from build123d import *

# Parameters (mm, degrees)
SKETCH_2_W      = 56
SKETCH_2_H      = 32
EXTRUDE_1_DEPTH = 3
SKETCH_3_W      = 56
SKETCH_3_H      = 32
SKETCH_3_W_2    = 25
SKETCH_3_H_2    = 14
EXTRUDE_2_DEPTH = 1
SKETCH_4_R      = 2.4
EXTRUDE_3_DEPTH = 5
SKETCH_6_W      = 56
SKETCH_6_H      = 2
EXTRUDE_4_DEPTH = 4
SKETCH_7_R      = 0.8
EXTRUDE_5_DEPTH = 5


with BuildPart() as part:
    # 草图2 → 凸台-拉伸1 (new body)
    with BuildSketch(Plane(origin=(0, 0, 0), x_dir=(1, 0, 0), z_dir=(0, 1, 0))):
        with Locations((6.832, -6.328)):
            Rectangle(SKETCH_2_W, SKETCH_2_H)
        Polygon((-20.168, -11.589207904), (-20.168, 4.317392289), (-20.168, 8.672), (33.832, 8.672), (33.832, -14.328), (20.832, -14.328), (20.832, -21.328), (-7.168, -21.328), (-7.168, -14.328), (-20.168, -14.328), align=None, mode=Mode.SUBTRACT)
    extrude(amount=EXTRUDE_1_DEPTH)

    # 草图3 → 凸台-拉伸2 (add)
    with BuildSketch(Plane(origin=(0, 3, 0), x_dir=(1, 0, 0), z_dir=(0, 1, 0))):
        with Locations((6.832, -6.328)):
            Rectangle(SKETCH_3_W, SKETCH_3_H)
        with Locations((6.832, -5.328)):
            Rectangle(SKETCH_3_W_2, SKETCH_3_H_2, mode=Mode.SUBTRACT)
    extrude(amount=EXTRUDE_2_DEPTH)

    # 草图4 → 凸台-拉伸3 (add)
    with BuildSketch(Plane(origin=(0, 0, 0), x_dir=(-1, 0, 0), z_dir=(0, -1, 0))):
        with Locations(Location((16.168, -18.328, 0), (0, 0, 270))):
            Circle(SKETCH_4_R)
        with Locations(Location((-29.832, -18.328, 0), (0, 0, 270))):
            Circle(SKETCH_4_R)
    extrude(amount=EXTRUDE_3_DEPTH)

    # 草图6 → 凸台-拉伸4 (add)
    with BuildSketch(Plane(origin=(0, 4, 0), x_dir=(-1, 0, 0), z_dir=(0, -1, 0))):
        with Locations((-6.832, 10.672)):
            Rectangle(SKETCH_6_W, SKETCH_6_H)
    extrude(amount=EXTRUDE_4_DEPTH)

    # 草图7 → 凸台-拉伸5 (add)
    with BuildSketch(Plane(origin=(0, 0, 0), x_dir=(-1, 0, 0), z_dir=(0, -1, 0))):
        with Locations(Location((-29.832, 10.172, 0), (0, 0, 270))):
            Circle(SKETCH_7_R)
        with Locations(Location((16.168, 10.172, 0), (0, 0, 270))):
            Circle(SKETCH_7_R)
    extrude(amount=EXTRUDE_5_DEPTH)


solid = part.part
Work out the finished part from the listing and answer in its coordinate system (mm). A direction names the side the tool comes from. Round coordinates to 2 decimals unless told otherwise and drop trailing zeros. Write each loop counter-clockwise with the first axis right and the second up, starting at its lowest first coordinate (ties: lowest second). Pieces come first, ordered by that corner, then holes. Notation, with made-up numbers: (67, 72.5) - (91, 72.5) arc R35 cw to (91, 109.5) - close; hole circle Ø1 at (49.5, -23.5). An arc over 180 degrees is marked (long way). Answer in a Markdown table with one row per item. Add a question column.
1. The mould has two halves that part along X. Classify faces 4 (the flat face through (33.832, 1, 3)), 5 (the flat face through (34.832, 2, 6)), 6 (the flat face through (-16, -5, -10)), 7 (the flat face through (-20.168, 1, 3)): +X half, -X half, draft (parallel to the pull), parting line (faces both ways), or undercut.
2. A cutting plane is placed at C-C, the plane y = 2. Determine the outline of the cut face in (x, z).
3. For faces 1 (the flat face through (20.832, 1, 18)), 2 (the flat face through (7, 2, -11.672)), 3 (the flat face through (6.7, 3.5, 12.328)), determine the directions among +Z, -Z, +X, -X, +Y, -Y from which every point of the face is accessible in a straight line to the end or side of a thin tool.
4. Find the intervals of material crossed by line 1 along Z through (x, y) = (30, 1); line 2 along X through (y, z) = (0.5, 15.5); line 3 along X through (y, z) = (0.5, 8.5), in increasing order. Write a range as from..to.
5. Given pin 1 (4 mm diameter, centred on x = 23.5, z = -3.5, fed in from -Y); pin 2 (17 mm diameter, centred on x = 13, z = 13, fed in from -Y), each flat-ended and moving along its own axis, determine where each tip first touches the part or whether it passes through.
6. A cutting plane is placed at D-D, the plane z = -4.5. Determine the outline of the cut face in (x, y), and give its area (3 significant figures).
7. A cutting plane is placed at B-B, the plane z = 3.5. Determine the outline of the cut face in (x, y).
8. A cutting plane is placed at A-A, the plane x = 0.5. Determine the outline of the cut face in (y, z), and give its area (3 significant figures).
Worked out:
| question | item | result |
|---|---|---|
| 1 | face 4 | undercut |
| 1 | face 5 | +X half |
| 1 | face 6 | draft |
| 1 | face 7 | undercut |
| 2 | outline | (-21.17, -11.67) - (34.83, -11.67) - (34.83, 22.33) - (-21.17, 22.33) - close; hole (-20.17, -8.67) - (33.83, -8.67) - (33.83, 14.33) - (20.83, 14.33) - (20.83, 21.33) - (-7.17, 21.33) - (-7.17, 14.33) - (-20.17, 14.33) - close |
| 3 | face 1 | -Y |
| 3 | face 2 | -Z, +X, -X, +Y, -Y |
| 3 | face 3 | +Y, -Y |
| 4 | line 1 | -11.67..-8.67, 14.33..22.33 |
| 4 | line 2 | -21.17..-7.17, 20.83..34.83 |
| 4 | line 3 | -21.17..-20.17, 33.83..34.83 |
| 5 | pin 1 | y = 3 |
| 5 | pin 2 | y = 0 |
| 6 | outline | (-21.17, 0) - (-20.17, 0) - (-20.17, 3) - (33.83, 3) - (33.83, 0) - (34.83, 0) - (34.83, 4) - (-21.17, 4) - close |
| 6 | area | 62.0 mm^2 |
| 7 | outline | (-21.17, 0) - (-20.17, 0) - (-20.17, 3) - (-5.67, 3) - (-5.67, 4) - (-21.17, 4) - close; (19.33, 3) - (33.83, 3) - (33.83, 0) - (34.83, 0) - (34.83, 4) - (19.33, 4) - close |
| 8 | outline | (0, -11.67) - (4, -11.67) - (4, -1.67) - (3, -1.67) - (3, -8.67) - (0, -8.67) - close; (0, 21.33) - (3, 21.33) - (3, 12.33) - (4, 12.33) - (4, 22.33) - (0, 22.33) - close |
| 8 | area | 32.0 mm^2 |
